Check sheet for the modelled part. Datum: model origin and axes. Units: mm. A direction names the side the tool comes from. Round coordinates to 2 decimals unless told otherwise and drop trailing zeros. Order: outer loops, then holes, each group sorted by start corner. A loop starts at its lowest first (then second) coordinate and runs counter-clockwise, first axis right, second up. Notation, with made-up numbers: M 41.25,80 L 46.25,80 A12 cw 46.25,96 Z; hole C -26.75,47 d5. An arc over 180 degrees is marked long. One line per item, written item: value. Start each with the question number.
(1) Cross-section at D-D, the plane y = 32. Enter the section's corners in (x, z).
(2) Release check for a two-part mould opening along X. For faces 5 (the face through (-25.14, 26.32, -39.1)), 6 (the face through (-13, 27, -3)), 7 (the face through (-13, 0, -20)), 8 (the face through (-13, 27, -37)) record: released by +X, released by -X, zero draft, split by the parting line, or undercut.
(3) Depth check by flat-ended pin: pin 1 Ø6 at (x, z) = (-16, -24.5) entering from +Y; pin 2 Ø4 at (y, z) = (23.5, -32) entering from +X; pin 3 Ø12 at (y, z) = (7, -7.5) entering from -X. Enter the tip coordinate at first touch or a pass-through.
(4) Thickness scan on L1, parallel to Z at x = -20, y = 22.5; L2, parallel to X at y = 29, z = -5.5; L3, parallel to Y at x = -11.5, z = -31. Record the ranges inside material, lowest first.
(5) Cross-section at C-C, the plane x = -15.5. Enter the section's corners in (y, z).
(6) Access from +Z, -Z, +X, -X, +Y, -Y to the whole of each face (thin tool, end or side, straight path). Record for faces 1 (the face through (-21.5, 27, -20)), 2 (the face through (2.03, 32.07, -18.5)), 3 (the face through (-12.86, 0.9, -0.86)), 4 (the face through (-27.97, 31.93, -18.5)).
(7) Cross-section at A-A, the plane z = -17. Enter the section's corners in (x, y).
(8) Cross-section at B-B, the plane y = 17. Enter the section's corners in (x, z), and give its area (3 significant figures).
from build123d import *

# Parameters (mm, degrees)
CROQUIS1_W              = 26
CROQUIS1_H              = 40
SALIENTE_EXTRUIR1_DEPTH = 50
CROQUIS2_W              = 17
CROQUIS2_H              = 34
CORTAR_EXTRUIR1_DEPTH   = 47
REDONDEO1_R             = 3
REDONDEO2_R             = 1
CROQUIS4_R              = 1.5
SALIENTE_EXTRUIR2_DEPTH = 4
SALIENTE_EXTRUIR3_START = 4
CROQUIS5_R              = 1.5
SALIENTE_EXTRUIR3_DEPTH = 4


with BuildPart() as part:
    # Croquis1 → Saliente-Extruir1 (new body)
    with BuildSketch(Plane(origin=(0, 0, 0), x_dir=(1, 0, 0), z_dir=(0, 1, 0))):
        with Locations((-13, 20)):
            Rectangle(CROQUIS1_W, CROQUIS1_H)
    extrude(amount=SALIENTE_EXTRUIR1_DEPTH)

    # Croquis2 → Cortar-Extruir1 (cut)
    with BuildSketch(Plane(origin=(0, 50, 0), x_dir=(1, 0, 0), z_dir=(0, 1, 0))):
        with Locations((-13, 20)):
            Rectangle(CROQUIS2_W, CROQUIS2_H)
    extrude(amount=-CORTAR_EXTRUIR1_DEPTH, mode=Mode.SUBTRACT)

    # Redondeo1
    redondeo1_edges = [part.edges().sort_by_distance(p)[0] for p in [
        (-13, 0, 0),
        (-26, 0, -20),
        (-13, 0, -40),
        (0, 0, -20),
        (0, 25, 0),
        (-26, 25, 0),
        (-26, 25, -40),
        (0, 25, -40),
    ]]
    fillet(redondeo1_edges, radius=REDONDEO1_R)

    # Redondeo2
    redondeo2_edges = [part.edges().sort_by_distance(p)[0] for p in [
        (-13, 50, -40),
        (-26, 50, -20),
        (-13, 50, 0),
        (0, 50, -20),
        (-25.121320344, 50, -0.878679656),
        (-0.878679656, 50, -0.878679656),
        (-0.878679656, 50, -39.121320344),
        (-25.121320344, 50, -39.121320344),
    ]]
    fillet(redondeo2_edges, radius=REDONDEO2_R)

    # Croquis4 → Saliente-Extruir2 (add)
    with BuildSketch(Plane.ZY.offset(26)):
        with Locations(Location((-20, 32, 0), (0, 0, 180))):
            Circle(CROQUIS4_R)
    extrude(amount=SALIENTE_EXTRUIR2_DEPTH)

    # Croquis5 → Saliente-Extruir3 (add)
    with BuildSketch(Plane(origin=(0, 0, 0), x_dir=(0, 0, -1), z_dir=(1, 0, 0)).offset(SALIENTE_EXTRUIR3_START)):
        with Locations((20, 32)):
            Circle(CROQUIS5_R)
    extrude(amount=-SALIENTE_EXTRUIR3_DEPTH)


solid = part.part
Values found:
1. outline: M -30,-21.5 L -26,-21.5 L -26,-37 A3 ccw -23,-40 L -3,-40 A3 ccw 0,-37 L 0,-21.5 L 4,-21.5 L 4,-18.5 L 0,-18.5 L 0,-3 A3 ccw -3,0 L -23,0 A3 ccw -26,-3 L -26,-18.5 L -30,-18.5 Z; hole M -21.5,-37 L -4.5,-37 L -4.5,-3 L -21.5,-3 Z
2. face 5: released by -X
2. face 6: undercut
2. face 7: zero draft
2. face 8: undercut
3. pin 1: y = 3
3. pin 2: x = 0
3. pin 3: x = -26
4. L1: -40 to -37, -3 to 0
4. L2: -26 to -21.5, -4.5 to 0
4. L3: 0 to 3
5. outline: M 0,-37 A3 ccw 3,-40 L 49,-40 A1 ccw 50,-39 L 50,-37 L 3,-37 L 3,-3 L 50,-3 L 50,-1 A1 ccw 49,0 L 3,0 A3 ccw 0,-3 Z
6. face 1: +Y
6. face 2: +X
6. face 3: +Z, +X, -X, -Y
6. face 4: -X
7. outline: M -26,3 A3 ccw -23,0 L -3,0 A3 ccw 0,3 L 0,49 A1 ccw -1,50 L -4.5,50 L -4.5,3 L -21.5,3 L -21.5,50 L -25,50 A1 ccw -26,49 Z
8. outline: M -26,-37 A3 ccw -23,-40 L -3,-40 A3 ccw 0,-37 L 0,-3 A3 ccw -3,0 L -23,0 A3 ccw -26,-3 Z; hole M -21.5,-37 L -4.5,-37 L -4.5,-3 L -21.5,-3 Z
8. area: 454 mm^2
